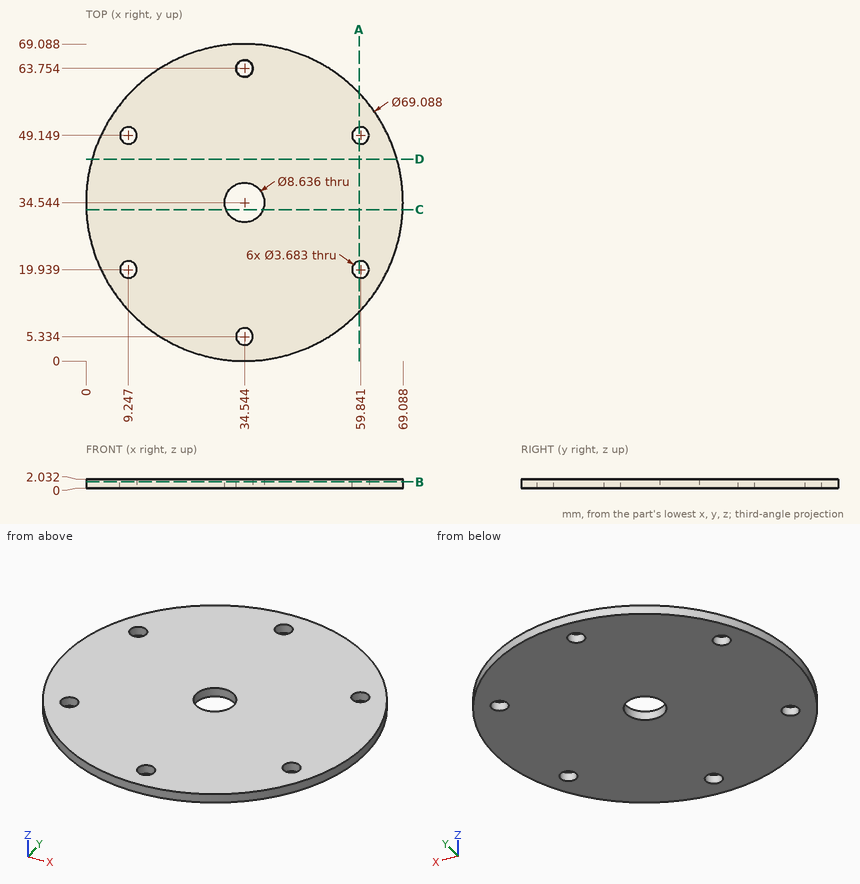
Could you check a few things on this drawing? It's one solid part, dimensions in mm from its lowest x, y, z. Coordinates: 2 decimals unless noted, no trailing zeros. Write each loop counter-clockwise with the first axis right and the second up, starting at its lowest first coordinate (ties: lowest second). Pieces come first, ordered by that corner, then holes. Notation, with made-up numbers: (22.5, 32.25) - (76.5, 32.25) arc R24 ccw to (76.5, 55.25) - close; hole circle Ø9 at (-38.5, 39). An arc over 180 degrees is marked (long way). Write item = value, one per line.
1) Suppose I cut it at D-D on y = 44. Please give me the cut outline in (x, z).
Result set:
outline = (1.32, 0) - (67.77, 0) - (67.77, 2.03) - (1.32, 2.03) - close
2) Suppose I cut it at B-B on z = 1.4. Please give me the cut outline in (x, y) (1 decimal).
Result set:
outline = circle Ø69.1 at (34.5, 34.5); hole circle Ø3.7 at (9.2, 19.9); hole circle Ø3.7 at (9.2, 49.1); hole circle Ø8.6 at (34.5, 34.5); hole circle Ø3.7 at (34.5, 5.3); hole circle Ø3.7 at (34.5, 63.8); hole circle Ø3.7 at (59.8, 19.9); hole circle Ø3.7 at (59.8, 49.1)
3) Will these pins go through, and if not, where does the flat tip stop? pin 1 Ø1 at (x, z) = (10.5, 1.5) entering from +Y; pin 2 Ø2 at (x, y) = (34.544, 5.334) entering from +Z.
Result set:
pin_1 = 59.82
pin_2 = through
4) Please list where these lines run through material, in increasing order: line 1 (Y direction, x = 9, z = 0.9) (1 decimal); line 2 (X direction, y = 20, z = 0.7); line 3 (Y direction, x = 59, z = 1.75). Write a range as [from, to].
Result set:
line_1 = [11.3, 18.1], [21.8, 47.3], [51, 57.8]
line_2 = [3.21, 7.41], [11.09, 58], [61.68, 65.88]
line_3 = [10.15, 18.3], [21.58, 47.51], [50.79, 58.94]
5) Suppose I cut it at A-A on x = 59.5. Please give me the cut outline in (y, z).
Result set:
outline = (10.66, 0) - (18.13, 0) - (18.13, 2.03) - (10.66, 2.03) - close; (21.75, 0) - (47.34, 0) - (47.34, 2.03) - (21.75, 2.03) - close; (50.96, 0) - (58.43, 0) - (58.43, 2.03) - (50.96, 2.03) - close
6) Suppose I cut it at C-C on y = 33. Please give me the cut outline in (x, z) (1 decimal), plus the area to 3 significant figures.
Result set:
outline = (0, 0) - (30.5, 0) - (30.5, 2) - (0, 2) - close; (38.6, 0) - (69.1, 0) - (69.1, 2) - (38.6, 2) - close
area = 124 mm2
